For this review, take the finished solid that the model builds, in its own axes (mm). Face numbers are marked on the shaded views. A direction names the side the tool comes from. Round coordinates to 2 decimals unless told otherwise and drop trailing zeros. Order: outer loops, then holes, each group sorted by start corner. A loop starts at its lowest first (then second) coordinate and runs counter-clockwise, first axis right, second up. Notation, with made-up numbers: (64, 51.25) - (95, 51.25) arc R15 cw to (95, 56.25) - close; hole circle Ø1 at (78.5, -27). An arc over 180 degrees is marked (long way). One line per question, with ' | ' between items.
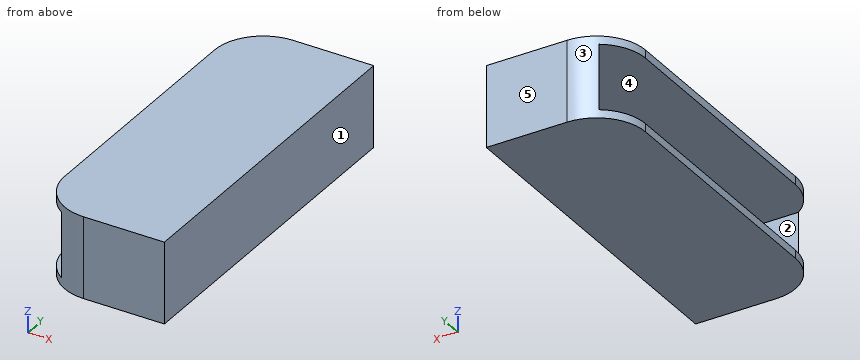
```python
from build123d import *

# Parameters (mm, degrees)
F0_W        = 39.7482234985
F0_H        = 105.248818174
F1_DEPTH    = 25
F2_T        = -2.5
F3_T1_DEPTH = 100


# Not quite as in the source:
# - a fillet or chamfer that OpenCascade refuses, or shapes differently, is made with other operations: its cross-section is extruded or revolved along the edge and cut away or added


with BuildPart() as f1:
    # F0 (on Top) → F1 (new body)
    with BuildSketch(Plane.XY):
        with Locations((1.5861960128, 22.0201415941)):
            Rectangle(F0_W, F0_H)
    extrude(amount=F1_DEPTH)

    # F2
    f2_openings = [f1.faces().sort_by_distance(p)[0] for p in [
        (-18.287916, 22.020142, 12.5),
    ]]
    offset(amount=F2_T, openings=f2_openings)

    # F3: fillet of radius 15 on 2 edges, made by hand

    # F3_s2 → F3_t1 (cut)
    with BuildSketch(Plane.XY.offset(-37.5)):
        with BuildLine():
            ThreePointArc((-3.2879157364, 74.6445506811), (-13.8945174542, 70.2511523989), (-18.2879157364, 59.6445506811))
            Line((-18.2879157364, 59.6445506811), (-18.2879157364, 74.6445506811))
            Line((-18.2879157364, 74.6445506811), (-3.2879157364, 74.6445506811))
        make_face()
        with BuildLine():
            ThreePointArc((-3.2879157364, -30.6042674929), (-13.8945174542, -26.2108692107), (-18.2879157364, -15.6042674929))
            Line((-18.2879157364, -15.6042674929), (-18.2879157364, -30.6042674929))
            Line((-18.2879157364, -30.6042674929), (-3.2879157364, -30.6042674929))
        make_face()
    extrude(amount=F3_T1_DEPTH, mode=Mode.SUBTRACT)


solid = f1.part
```
(1) We need section A-A on x = 13. State the section outline as (y, z) points.
Output values:
outline: (-30.6, 0) - (74.64, 0) - (74.64, 25) - (-30.6, 25) - close; hole (-28.1, 2.5) - (72.14, 2.5) - (72.14, 22.5) - (-28.1, 22.5) - close
(2) Insertion check: pin 1 (1.5 mm diameter, centred on y = 55, z = 19, fed in from -X); pin 2 (2 mm diameter, centred on x = -11.5, z = 6, fed in from -Y). Each pin has a flat end and moves straight along its axis. Give the tip position at first contact, or say it passes through.
Output values:
pin 1: x = 18.96 | pin 2: y = -28.76
(3) We need section B-B on y = 14.5. State the section outline as (x, z) points, plus the area to 3 significant figures.
Output values:
outline: (-18.29, 0) - (21.46, 0) - (21.46, 25) - (-18.29, 25) - (-18.29, 22.5) - (18.96, 22.5) - (18.96, 2.5) - (-18.29, 2.5) - close | area: 249 mm^2
(4) We need section D-D on x = -7. State the section outline as (y, z) points, plus the area to 3 significant figures.
Output values:
outline: (-30.14, 0) - (74.18, 0) - (74.18, 25) - (-30.14, 25) - close; hole (-28.1, 2.5) - (72.14, 2.5) - (72.14, 22.5) - (-28.1, 22.5) - close | area: 603 mm^2
(5) For probe 1 along Z at (x, y) = (-5.5, 58); probe 2 along Y at (x, z) = (0.5, 6.75); probe 3 along X at (y, z) = (-7.5, 15), list the stretches that pass through material, from the lowest coordinate up. Write a range as [from, to].
Output values:
probe 1: [0, 2.5], [22.5, 25] | probe 2: [-30.6, -28.1], [72.14, 74.64] | probe 3: [18.96, 21.46]
(6) Mouldability with a two-part tool opening along Y and no side actions: class the marked faces 1, 2 and 3 as released by +Y, released by -Y, zero draft, split by the parting line, or undercut.
Output values:
face 1: zero draft | face 2: undercut | face 3: released by +Y
(7) For the marked faces 4 and 5, list the 3-axis set-ups (+Z, -Z, +X, -X, +Y, -Y) from which the entire face can be reached by the end or side of a thin tool; tool diameter is ignored.
Output values:
face 4: -X | face 5: +Z, -Z, +X, -X, +Y
(8) We need section C-C on z = 4.75. State the section outline as (x, y) points.
Output values:
outline: (-11.58, -28.1) arc R15 ccw to (-3.29, -30.6) - (21.46, -30.6) - (21.46, 74.64) - (-3.29, 74.64) arc R15 ccw to (-11.58, 72.14) - (18.96, 72.14) - (18.96, -28.1) - close
